The drawing under review shows one solid part. Ordinate dimensions are in mm from its lowest x, y, z. A direction names the side the tool comes from. Coordinates: 2 decimals unless noted, no trailing zeros. Write each loop counter-clockwise with the first axis right and the second up, starting at its lowest first coordinate (ties: lowest second). Pieces come first, ordered by that corner, then holes. Notation, with made-up numbers: (43.5, 24) -> (76.5, 24) arc R29 cw to (76.5, 44) -> close; hole circle Ø9 at (29, 38). An arc over 180 degrees is marked (long way). One line per question, with ' | ' between items. Start each with the question number.
Q1. Add section D-D on y = 5. State the section outline as (x, z) points, and give its area (3 significant figures).
Q2. For P1, Ø1, axis at y = 3, z = 2, coming from the +X side (1 decimal); P2, Ø2, axis at x = 15, y = 4.5, coming from the -Z side; P3, Ø1.5, axis at y = 2, z = 3.5, coming from the -X side, all flat-tipped, find the tip position at first contact; note any pin that passes through.
Q3. For the marked faces 1, 2 and 3, list the 3-axis set-ups (+Z, -Z, +X, -X, +Y, -Y) from which the entire face can be reached by the end or side of a thin tool; tool diameter is ignored.
Q4. Wall thickness on probe 1 along X at (y, z) = (2, 9); probe 2 along Z at (x, y) = (9, 3); probe 3 along Z at (x, y) = (9, 7): over which ranges is each line inside the solid? List them lowest first.
Q5. Add section C-C on z = 10.25. State the section outline as (x, y) points, and give its area (3 significant figures).
Q6. Draft analysis for pull direction X (two halves, no side actions). For the marked faces 4, 5, 6 and 7, state which applies: pulls with the +X half, pulls with the -X half, needs draft (parallel to the pull), parting line crosses it, or undercut.
Q7. Add section A-A on x = 9. State the section outline as (y, z) points, and give its area (3 significant figures).
Q8. Add section B-B on y = 3. State the section outline as (x, z) points.
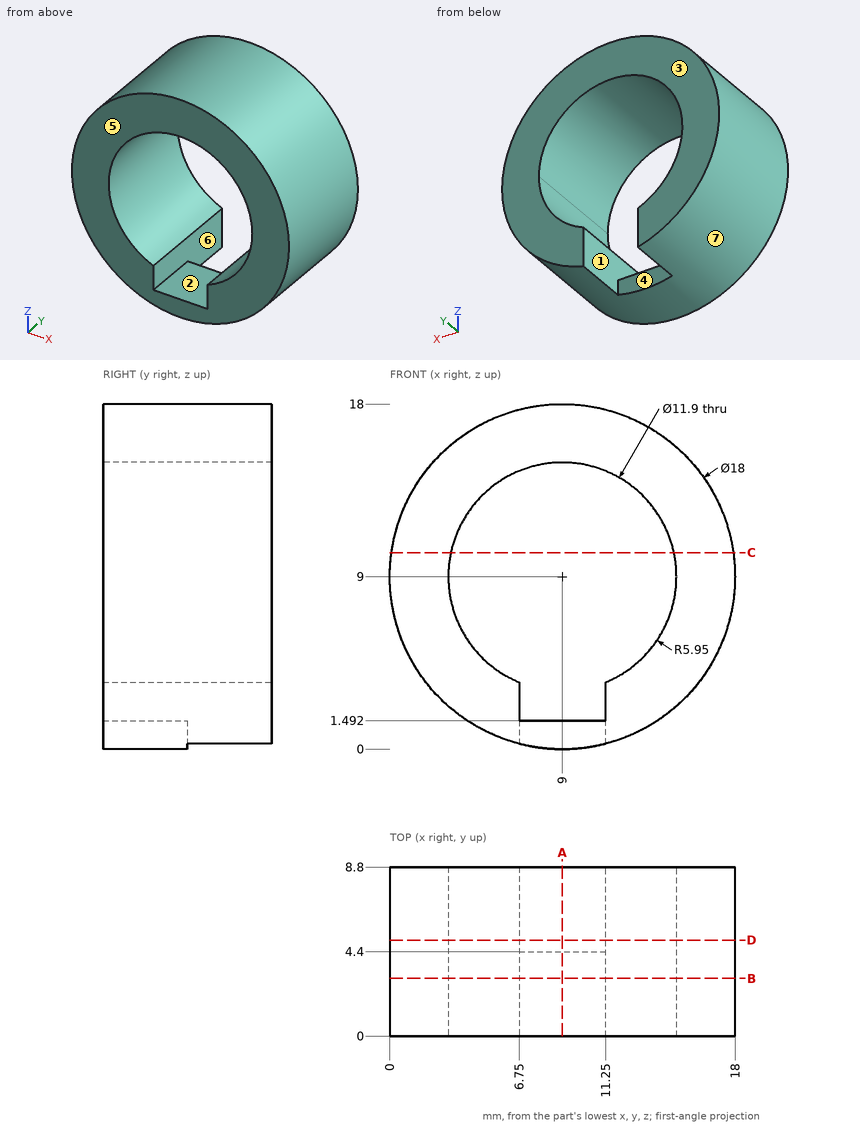
Output values:
1) outline: (6.75, 0.29) -> (6.75, 3.49) arc R5.95 cw (long way) to (11.25, 3.49) -> (11.25, 0.29) arc R9 ccw (long way) to start | area: 129 mm2
2) P1: stops at x = 15.2 | P2: stops at z = 1.52 | P3: stops at x = 1.36
3) face 1: +Y | face 2: +Y, -Y | face 3: +Z, -Z, +X, -X, +Y
4) probe 1: x = 0 to 3.05, 14.95 to 18 | probe 2: z = 0 to 1.49, 14.95 to 18 | probe 3: z = 14.95 to 18
5) outline: (0.09, 0) -> (3.18, 0) -> (3.18, 8.8) -> (0.09, 8.8) -> close; (14.82, 0) -> (17.91, 0) -> (17.91, 8.8) -> (14.82, 8.8) -> close | area: 54.5 mm2
6) face 4: undercut | face 5: needs draft | face 6: undercut | face 7: parting line crosses it
7) outline: (0, 0) -> (4.4, 0) -> (4.4, 1.49) -> (0, 1.49) -> close; (0, 14.95) -> (8.8, 14.95) -> (8.8, 18) -> (0, 18) -> close | area: 33.4 mm2
8) outline: circle Ø18 at (9, 9); hole (6.75, 1.49) -> (11.25, 1.49) -> (11.25, 3.49) arc R5.95 ccw (long way) to (6.75, 3.49) -> close
